The listing builds one solid part. Answer for the finished solid, in the listing's coordinates (mm). A direction names the side the tool comes from. Round coordinates to 2 decimals unless told otherwise and drop trailing zeros. Loops run counter-clockwise (first coordinate to the right, second up) from the corner with the lowest first, then second, coordinate; pieces in that order, holes last. Notation, with made-up numbers: (41, -7) -> (56, -7) arc R23 cw to (56, 15) -> close; hole circle Ø6 at (67.25, 1.5). An arc over 180 degrees is marked (long way). Answer in a Markdown table with one row per item. Add a question column.
Autodesk Inventor part; units mm, degrees
ref_plane "YZ Plane" through (0, 0, 0) normal (1, 0, 0) x (0, 1, 0)
ref_plane "XZ Plane" through (0, 0, 0) normal (0, 1, 0) x (-1, 0, 0)
ref_plane "XY Plane" through (0, 0, 0) normal (0, 0, 1) x (1, 0, 0)
sketch "Sketch1" plane through (0, 0, 0) normal (1, 0, 0) x (0, 1, 0)
  line L0 (-10, 4) -> (10, 4)
  line L1 (10, 4) -> (10, -4)
  line L2 (10, -4) -> (-10, -4)
  line L3 (-10, -4) -> (-10, 4)
  line L4 (-10, 4) -> (10, -4) construction
  line L5 (10, 4) -> (-10, -4) construction
  point P0 (0, 0)
  dimension "d0" = 8
  dimension "d1" = 20
extrude "Extrusion1" add sketch "Sketch1" along normal blind 39.9
sketch "Sketch2" plane through (39.9, 0, 0) normal (1, 0, 0) x (0, 0, -1)
  line L0 (-4, 10) -> (-4, -10)
  line L1 (-4, 4.5) -> (0.5, 4.5)
  line L2 (0.5, 4.5) -> (0.5, -4.5)
  line L3 (0.5, -4.5) -> (-4, -4.5)
  line L4 (-4, -4.5) -> (-4, 4.5)
  point P0 (0, 0)
  dimension "d4" = 9
  dimension "d5" = 4.5
  dimension "d6" = 4.5
extrude "Extrusion2" cut sketch "Sketch2" against normal blind 39.9
sketch "Sketch3" plane through (0, -10, -4) normal (0, 0, -1) x (-1, 0, 0)
  line L0 (0, 20) -> (0, 0)
  line L1 (0, 20) -> (-39.9, 20)
  line L2 (-39.9, 0) -> (-39.9, 20)
  line L3 (0, 0) -> (-39.9, 0)
  point P0 (0, 10)
  point P1 (-27.95, 17.5)
  point P2 (-27.95, 2.5)
  point P3 (-11.95, 2.5)
  point P4 (-11.95, 17.5)
  dimension "d9" = 16
  dimension "d10" = 39.9
  dimension "d11" = 11.95
  dimension "d12" = 15
  dimension "d13" = 7.5
hole "Hole1" at (27.95, 7.5, -4) at (27.95, -7.5, -4) at (11.95, -7.5, -4) at (11.95, 7.5, -4) direction (0, 0, 1) diameter 2.459 depth 5 tip angle 118
properties part number "MGN9H" material "Stainless Steel AISI 440C, Welded"
Item 1: The mould has two halves that part along X. Classify faces 1 (the conical face through (12.16, 7.47, 1.61)), 2 (the flat face through (0, 0, -1)), 3 (the flat face through (20, 4.5, 2)): +X half, -X half, draft (parallel to the pull), parting line (faces both ways), or undercut.
Item 2: Section D-D, the plane y = 0 is taken. Write down the section's boundary in (x, z), and give its area (3 significant figures).
Item 3: For faces 4 (the cylindrical face through (13.04, 8.07, -1.46)), 5 (the flat face through (20, 0, -0.5)), 6 (the flat face through (20, 0, -4)), determine the directions among +Z, -Z, +X, -X, +Y, -Y from which every point of the face is accessible in a straight line to the end or side of a thin tool.
Item 4: Section A-A, the plane z = 3.5 is taken. Write down the section's boundary in (x, y), and give its area (3 significant figures).
Item 5: Section C-C, the plane z = -1.5 is taken. Write down the section's boundary in (x, y), and give its area (3 significant figures).
Item 6: Section B-B, the plane x = 23 is taken. Write down the section's boundary in (y, z), and give its area (4 significant figures).
Item 7: Flat-ended cylindrical pins translate along their axes: P1, Ø1.5, axis at x = 11.95, y = 7.5, coming from the -Z side; P2, Ø5, axis at x = 14.5, y = -1, coming from the +Z side. Find the tip coordinate at first contact, or state that the pin passes through.
Item 8: Consider L1, parallel to Y at x = 27.95, z = -1.4; L2, parallel to X at y = 7.5, z = -2.5; L3, parallel to Y at x = 11.95, z = -0.45. Determine where each line is inside the solid, lowest interval first. Write a range as from..to.
Here are the results:
| question | item | result |
|---|---|---|
| 1 | face 1 | undercut |
| 1 | face 2 | -X half |
| 1 | face 3 | draft |
| 2 | outline | (0, -4) -> (39.9, -4) -> (39.9, -0.5) -> (0, -0.5) -> close |
| 2 | area | 140 mm² |
| 3 | face 4 | -Z |
| 3 | face 5 | +Z, +X, -X |
| 3 | face 6 | -Z, +X, -X, +Y, -Y |
| 4 | outline | (0, -10) -> (39.9, -10) -> (39.9, -4.5) -> (0, -4.5) -> close; (0, 4.5) -> (39.9, 4.5) -> (39.9, 10) -> (0, 10) -> close |
| 4 | area | 439 mm² |
| 5 | outline | (0, -10) -> (39.9, -10) -> (39.9, 10) -> (0, 10) -> close; hole circle Ø2.46 at (11.95, -7.5); hole circle Ø2.46 at (11.95, 7.5); hole circle Ø2.46 at (27.95, -7.5); hole circle Ø2.46 at (27.95, 7.5) |
| 5 | area | 779 mm² |
| 6 | outline | (-10, -4) -> (10, -4) -> (10, 4) -> (4.5, 4) -> (4.5, -0.5) -> (-4.5, -0.5) -> (-4.5, 4) -> (-10, 4) -> close |
| 6 | area | 119.5 mm² |
| 7 | P1 | stops at z = 1.29 |
| 7 | P2 | stops at z = -0.5 |
| 8 | L1 | y = -10..-8.73, -6.27..6.27, 8.73..10 |
| 8 | L2 | x = 0..10.72, 13.18..26.72, 29.18..39.9 |
| 8 | L3 | y = -10..-8.73, -6.27..-4.5, 4.5..6.27, 8.73..10 |
